Geometry check sheet. Reference: the model listing, model coordinates, mm. A direction names the side the tool comes from. Coordinates: 2 decimals unless noted, no trailing zeros. Write each loop counter-clockwise with the first axis right and the second up, starting at its lowest first coordinate (ties: lowest second). Pieces come first, ordered by that corner, then holes. Notation, with made-up numbers: M 56,27 L 80,27 A6 cw 80,34 Z; hole C 87.25,3 d8. An arc over 180 degrees is marked long. Answer as a JSON object with one key per item and string values. Group by question number.
```python
from build123d import *

# Parameters (mm, degrees)
BASEHEADSKE_R   = 2.25
BASEHEAD_DEPTH  = 2.5
CUTSOCKET_DEPTH = 1.1
FILLET1_R       = 0.1
FILLET2_R       = 0.25


with BuildPart() as part:
    # BaseHeadSke → BaseHead (new body)
    with BuildSketch(Plane(origin=(0, 0, 0), x_dir=(0, 0, -1), z_dir=(1, 0, 0))):
        Circle(BASEHEADSKE_R)
    extrude(amount=BASEHEAD_DEPTH)

    # BodySke → BaseBody (revolve)
    with BuildSketch(Plane.XY, mode=Mode.PRIVATE) as basebody_sk:
        Polygon((0, 0), (14.5, 0), (14.5, 0.9965), (14.2465, 1.25), (0, 1.25), align=None)
    revolve(basebody_sk.sketch.rotate(Axis((0, 0, 0), (1, 0, 0)), 90), axis=Axis((0, 0, 0), (1, 0, 0)))

    # CutSocketSke → CutSocket (cut)
    with BuildSketch(Plane(origin=(0, 0, 0), x_dir=(0, 0, -1), z_dir=(1, 0, 0))):
        Polygon((0, 1.154700538), (-1, 0.577350269), (-1, -0.577350269), (0, -1.154700538), (1, -0.577350269), (1, 0.577350269), align=None)
    extrude(amount=CUTSOCKET_DEPTH, mode=Mode.SUBTRACT)

    # CutHoleSke → CutHole (revolve, cut)
    with BuildSketch(Plane.XY, mode=Mode.PRIVATE) as cuthole_sk:
        Polygon((0, 1), (1.65, 1), (2.227350269, 0), (0, 0), align=None)
    revolve(cuthole_sk.sketch.rotate(Axis((0, 0, 0), (1, 0, 0)), 90), axis=Axis((0, 0, 0), (1, 0, 0)), mode=Mode.SUBTRACT)

    # Fillet1
    fillet1_edges = [part.edges().sort_by_distance(p)[0] for p in [
        (2.5, 0, -1.25),
    ]]
    fillet(fillet1_edges, radius=FILLET1_R)

    # Fillet2
    fillet2_edges = [part.edges().sort_by_distance(p)[0] for p in [
        (0, 0, 2.25),
    ]]
    fillet(fillet2_edges, radius=FILLET2_R)


solid = part.part
```
1) Set-up check for faces 1 (the cylindrical face through (1.379, 0.976, -0.217)), 2 (the flat face through (14.5, 0, 0)), 3 (the flat face through (2.5, -1.5, -0.5)): record each of +Z, -Z, +X, -X, +Y, -Y from which the full face is reachable in a straight line by a thin tool's end or side.
2) Draft check along Z on faces 4 (the flat face through (0, -1, -1)), 5 (the flat face through (0.5, 0, 1)), 6 (the flat face through (0.54, -0.86, 0.51)), 7 (the cylindrical face through (1.36, 2.23, 0.29)). Enter one of: +Z half, -Z half, draft (parallel to the pull), parting line (faces both ways), or undercut.
3) Go/stop test with flat-tipped pins: pin 1 Ø1.5 at (x, y) = (11.5, 1.5) entering from -Z; pin 2 Ø1 at (x, y) = (3.5, -1.5) entering from +Z. Record where each tip stops, or that it passes through.
4) Section check A-A (x = 4.25). Record the cut outline in (y, z), then the cut area to 3 significant figures.
5) Material ranges on probe 1 along Y at (x, z) = (1.55, 0); probe 2 along X at (y, z) = (-0.2, -1.65); probe 3 along Y at (x, z) = (6.5, 0.9), recorded low to high. Write a range as [from, to].
Entries:
{
 "1": {"face 1": "-X", "face 2": "+Z, -Z, +X, +Y, -Y", "face 3": "+X"},
 "2": {"face 4": "draft", "face 5": "undercut", "face 6": "undercut", "face 7": "parting line"},
 "3": {"pin 1": "z = -1", "pin 2": "z = 0.75"},
 "4": {"outline": "C 0,0 d2.5", "area": "4.91 mm^2"},
 "5": {"probe 1": "[-2.25, -1], [1, 2.25]", "probe 2": "[0, 2.5]", "probe 3": "[-0.87, 0.87]"}
}
